Verification items for the finished model (mm, model axes). Face numbers are marked on the shaded views. A direction names the side the tool comes from. Give positions to 0.01 mm unless a question says otherwise; leave off trailing zeros. Write each loop counter-clockwise with the first axis right and the second up, starting at its lowest first coordinate (ties: lowest second). Pieces come first, ordered by that corner, then holes. Notation, with made-up numbers: M 84.5,65 L 118.5,65 A29 cw 118.5,92 Z; hole C 54,15.5 d11. An arc over 180 degrees is marked long. Answer as a JSON object with one key per item and string values.
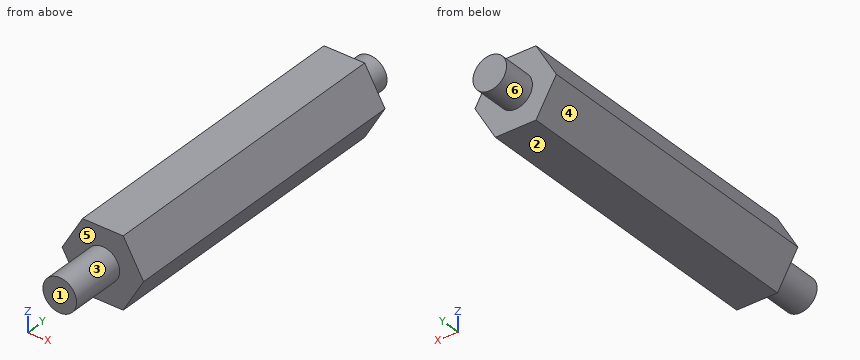
```python
from build123d import *

# Parameters (mm, degrees)
F0_R     = 1.5
F1_DEPTH = 14
F2_DEPTH = 19
F3_DEPTH = 17


with BuildPart() as f1:
    # F0 (on Front) → F1 (new body, symmetric)
    with BuildSketch(Plane.XZ):
        Polygon((-2.879062, 0), (-1.060408, -3.15), (2.576898, -3.15), (4.395552, 0), (2.576898, 3.15), (-1.060408, 3.15), align=None)
        with Locations((0.758245, 0)):
            Circle(F0_R, mode=Mode.SUBTRACT)
    extrude(amount=F1_DEPTH, both=True)

    # F0 (on Front) → F2 (join)
    with BuildSketch(Plane.XZ):
        with Locations((0.758245, 0)):
            Circle(F0_R)
    extrude(amount=F2_DEPTH)

    # F0 (on Front) → F3 (join)
    with BuildSketch(Plane.XZ):
        with Locations((0.758245, 0)):
            Circle(F0_R)
    extrude(amount=-F3_DEPTH)


solid = f1.part
```
1) Access from +Z, -Z, +X, -X, +Y, -Y to the whole of each face (thin tool, end or side, straight path). Record for the marked faces 4, 5 and 6.
Completed:
{"face 4": "-Z, -X, +Y, -Y", "face 5": "-Y", "face 6": "+Y"}
2) Go/stop test with a flat-tipped pin: pin 1 (3 mm diameter, centred on y = -13, z = -2, fed in from -X). Record where the tip stops, or that it passes through.
Completed:
{"pin 1": "stops at x = -2.59"}
3) Section check A-A on z = 0.75. Record the boundary of the cut face in (x, y), and give its area (3 significant figures).
Completed:
{"outline": "M -2.45,-14 L -0.54,-14 L -0.54,-19 L 2.06,-19 L 2.06,-14 L 3.96,-14 L 3.96,14 L 2.06,14 L 2.06,17 L -0.54,17 L -0.54,14 L -2.45,14 Z", "area": "200 mm2"}
4) Thickness scan on L1, parallel to Y at x = 0, z = 2.25; L2, parallel to Z at x = -0.5, y = -15.5; L3, parallel to Z at x = 3, y = -11. Record the ranges inside material, lowest first.
Completed:
{"L1": "y = -14 to 14", "L2": "z = -0.82 to 0.82", "L3": "z = -2.42 to 2.42"}
5) Section check D-D on y = 14.5. Record the boundary of the cut face in (x, z), and give its area (3 significant figures).
Completed:
{"outline": "C 0.76,0 d3", "area": "7.07 mm2"}
6) Section check B-B on x = 1.25. Record the boundary of the cut face in (y, z).
Completed:
{"outline": "M -19,-1.42 L -14,-1.42 L -14,-3.15 L 14,-3.15 L 14,-1.42 L 17,-1.42 L 17,1.42 L 14,1.42 L 14,3.15 L -14,3.15 L -14,1.42 L -19,1.42 Z"}
7) Release check for a two-part mould opening along Z. For the marked faces 1, 2 and 3 record: pulls with the +Z half, pulls with the -Z half, needs draft (parallel to the pull), parting line crosses it, or undercut.
Completed:
{"face 1": "needs draft", "face 2": "pulls with the -Z half", "face 3": "parting line crosses it"}
8) Section check C-C on y = -1. Record the boundary of the cut face in (x, z), and give its area (3 significant figures).
Completed:
{"outline": "M -2.88,0 L -1.06,-3.15 L 2.58,-3.15 L 4.4,0 L 2.58,3.15 L -1.06,3.15 Z", "area": "34.4 mm2"}
